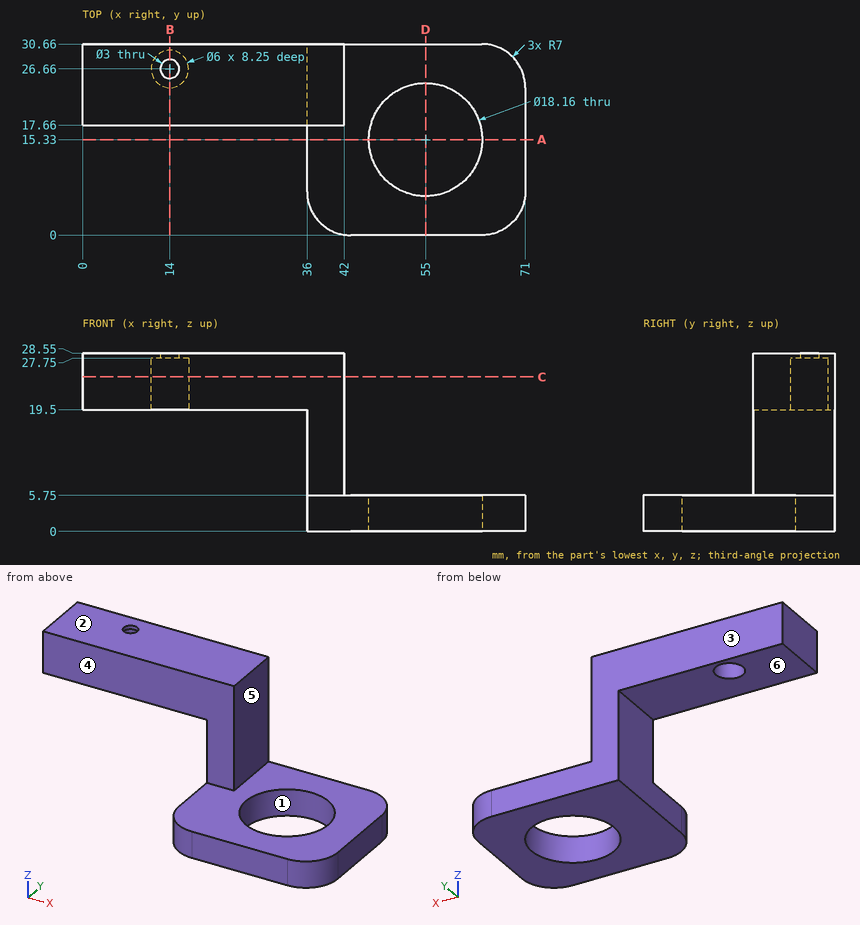
Source: three-view drawing plus pictorial views. Frame: mm from the lowest corner of the part. A direction names the side the tool comes from. Coordinates: 2 decimals unless noted, no trailing zeros. Order: outer loops, then holes, each group sorted by start corner. A loop starts at its lowest first (then second) coordinate and runs counter-clockwise, first axis right, second up.
1) First-contact query: P1, Ø3, axis at y = 25.5, z = 24, coming from the +X side; P2, Ø6.5, axis at x = 14.5, y = 25, coming from the -Z side; P3, Ø10, axis at y = 14.5, z = 11, coming from the -X side. Flat tips, straight axial feed; report the tip coordinate or a pass-through.
Result sheet:
P1: stops at x = 42
P2: stops at z = 19.5
P3: stops at x = 36
2) Section A-A (y = 15.33). Return loops of the section in (x, z), then the cut area to 3 significant figures.
Result sheet:
outline: (36, 0) - (45.92, 0) - (45.92, 5.75) - (36, 5.75) - close; (64.08, 0) - (71, 0) - (71, 5.75) - (64.08, 5.75) - close
area: 96.8 mm2
3) Section B-B (x = 14). Return loops of the section in (y, z).
Result sheet:
outline: (17.66, 19.5) - (23.66, 19.5) - (23.66, 27.75) - (25.16, 27.75) - (25.16, 28.55) - (17.66, 28.55) - close; (28.16, 27.75) - (29.66, 27.75) - (29.66, 19.5) - (30.66, 19.5) - (30.66, 28.55) - (28.16, 28.55) - close
4) Draft query along Y for the marked faces 1, 2 and 3. Return one class per face: released by +Y, released by -Y, zero draft, split by the parting line, or undercut.
Result sheet:
face 1: undercut
face 2: zero draft
face 3: released by +Y
5) Section C-C (z = 24.75). Return loops of the section in (x, y).
Result sheet:
outline: (0, 17.66) - (42, 17.66) - (42, 30.66) - (0, 30.66) - close; hole circle Ø6 at (14, 26.66)
6) Section D-D (x = 55). Return loops of the section in (y, z), then the cut area to 3 significant figures.
Result sheet:
outline: (0, 0) - (6.25, 0) - (6.25, 5.75) - (0, 5.75) - close; (24.41, 0) - (30.66, 0) - (30.66, 5.75) - (24.41, 5.75) - close
area: 71.9 mm2
7) Ray query, probe 1 along X at (y, z) = (15.33, 2.7); probe 2 along Y at (x, z) = (14, 22.5); probe 3 along Y at (x, z) = (14, 28.15). Return the intervals inside material, ascending.
Result sheet:
probe 1: x = 36 to 45.92, 64.08 to 71
probe 2: y = 17.66 to 23.66, 29.66 to 30.66
probe 3: y = 17.66 to 25.16, 28.16 to 30.66
8) Set-up query: the marked faces 4, 5 and 6. Return all of +Z, -Z, +X, -X, +Y, -Y with unobstructed straight access to the full face (end or side cutting, diameter ignored); none if empty.
Result sheet:
face 4: +Z, +X, -X, -Y
face 5: +Z, +X, +Y, -Y
face 6: -Z, -X, +Y, -Y
